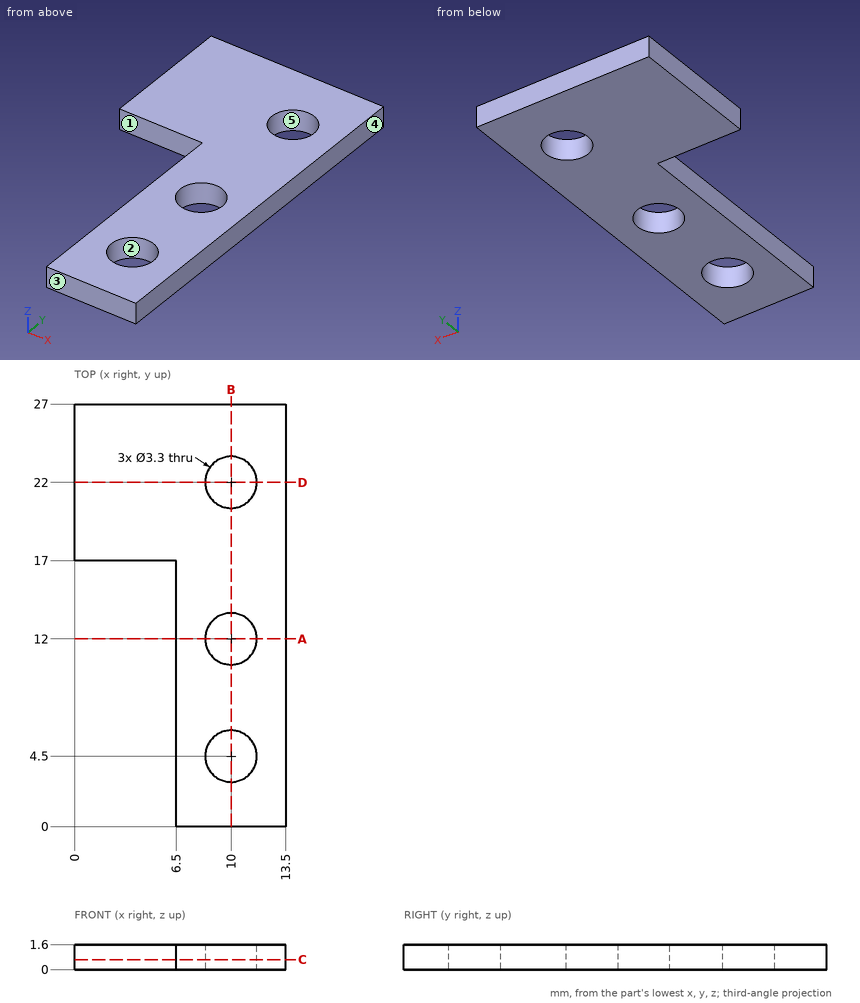
Could you check a few things on this drawing? It's one solid part, dimensions in mm from its lowest x, y, z. A direction names the side the tool comes from. Coordinates: 2 decimals unless noted, no trailing zeros. Loops run counter-clockwise (first coordinate to the right, second up) from the corner with the lowest first, then second, coordinate; pieces in that order, holes last.
1. For the marked faces 1 and 2, which set-ups out of +Z, -Z, +X, -X, +Y, -Y let a thin tool reach every point of the face, with its end or its side?
2. Imagine slicing it at D-D (y = 22). Please give me the cut outline in (x, z).
3. Imagine slicing it at C-C (z = 0.65). Please give me the cut outline in (x, y).
4. We'd pull the mould along X, two halves only. Please class the marked faces 3, 4 and 5: released by +X, released by -X, zero draft, split by the parting line, or undercut.
5. I need wall thicknesses on L1, parallel to Y at x = 10, z = 1.3; L2, parallel to Y at x = 9.25, z = 1.4; L3, parallel to X at y = 15, z = 0.6. Which ranges of each line are inside material? Lowest first, please.
6. Imagine slicing it at B-B (x = 10). Please give me the cut outline in (y, z).
7. Imagine slicing it at A-A (y = 12). Please give me the cut outline in (x, z), and give its area (3 significant figures).
Computed values:
1. face 1: +Z, -Z, -X, -Y
1. face 2: +Z, -Z
2. outline: (0, 0) - (8.35, 0) - (8.35, 1.6) - (0, 1.6) - close; (11.65, 0) - (13.5, 0) - (13.5, 1.6) - (11.65, 1.6) - close
3. outline: (0, 17) - (6.5, 17) - (6.5, 0) - (13.5, 0) - (13.5, 27) - (0, 27) - close; hole circle Ø3.3 at (10, 4.5); hole circle Ø3.3 at (10, 12); hole circle Ø3.3 at (10, 22)
4. face 3: zero draft
4. face 4: released by +X
4. face 5: undercut
5. L1: y = 0 to 2.85, 6.15 to 10.35, 13.65 to 20.35, 23.65 to 27
5. L2: y = 0 to 3.03, 5.97 to 10.53, 13.47 to 20.53, 23.47 to 27
5. L3: x = 6.5 to 13.5
6. outline: (0, 0) - (2.85, 0) - (2.85, 1.6) - (0, 1.6) - close; (6.15, 0) - (10.35, 0) - (10.35, 1.6) - (6.15, 1.6) - close; (13.65, 0) - (20.35, 0) - (20.35, 1.6) - (13.65, 1.6) - close; (23.65, 0) - (27, 0) - (27, 1.6) - (23.65, 1.6) - close
7. outline: (6.5, 0) - (8.35, 0) - (8.35, 1.6) - (6.5, 1.6) - close; (11.65, 0) - (13.5, 0) - (13.5, 1.6) - (11.65, 1.6) - close
7. area: 5.92 mm2
